```python
from build123d import *

# Parameters (mm, degrees)
SKETCH_1_R            = 12
EXTRUDE_1_DEPTH       = 55
CUT_EXTRUDE_START     = 19.5
SKETCH_2_OUTSIDE_W    = 38.926
SKETCH_2_OUTSIDE_H    = 38.926
SKETCH_2_OUTSIDE_R    = 10
CUT_EXTRUDE_1_DEPTH   = 3
SKETCH_3_R            = 11.5
EXTRUDE_2_DEPTH       = 18
SKETCH_4_OUTSIDE_W    = 42.1
SKETCH_4_OUTSIDE_H    = 42.1
SKETCH_4_OUTSIDE_R    = 11
CUT_EXTRUDE_2_DEPTH   = 2.5
SKETCH_5_R            = 10
EXTRUDE_3_DEPTH       = 16
SKETCH_6_OUTSIDE_W    = 45.05
SKETCH_6_OUTSIDE_H    = 45.05
SKETCH_6_OUTSIDE_R    = 9.5
CUT_EXTRUDE_3_DEPTH   = 2.5
SKETCH_7_R            = 9.5
EXTRUDE_4_DEPTH       = 28
SKETCH_9_R            = 10
EXTRUDE_6_DEPTH       = 15
SKETCH_10_R           = 10
EXTRUDE_7_DEPTH       = 24
SKETCH_11_OUTSIDE_W   = 57.93
SKETCH_11_OUTSIDE_H   = 57.93
SKETCH_11_OUTSIDE_R   = 9
CUT_EXTRUDE_4_DEPTH   = 11
CUT_EXTRUDE_START_2   = -21.5
SKETCH_12_OUTSIDE_W   = 57.93
SKETCH_12_OUTSIDE_H   = 57.93
SKETCH_12_OUTSIDE_R   = 9
CUT_EXTRUDE_5_DEPTH   = 2.5
CUT_EXTRUDE_8_DEPTH   = 157.920361967
CUT_EXTRUDE_START_3   = 8
CUT_EXTRUDE_9_DEPTH   = 149.920361967
CUT_EXTRUDE_START_4   = 8.5
CUT_EXTRUDE_10_DEPTH  = 149.420361967
F_2_0MM_1_D           = 2
F_2_0MM_1_DEPTH       = 5
F_2_0MM_1_CSINK_D     = 5
F_2_0MM_1_CSINK_ANGLE = 60
F_2_0MM_1_TIP         = 0.600860619
F_2_0MM_4_D           = 2
F_2_0MM_4_DEPTH       = 5
F_2_0MM_4_CSINK_D     = 5
F_2_0MM_4_CSINK_ANGLE = 60
F_2_0MM_4_TIP         = 0.600860619


# Read off the part's stored shape, not the designer's step: M20 机械螺纹 螺柱1
with BuildPart() as part:
    # 草图1 → 凸台-拉伸1 (new body)
    with BuildSketch(Plane.XY):
        Circle(SKETCH_1_R)
    extrude(amount=EXTRUDE_1_DEPTH)

    # 草图2 outside → 切除-拉伸1 (cut)
    with BuildSketch(Plane.XY.offset(CUT_EXTRUDE_START)):
        Rectangle(SKETCH_2_OUTSIDE_W, SKETCH_2_OUTSIDE_H)
        Circle(SKETCH_2_OUTSIDE_R, mode=Mode.SUBTRACT)
    extrude(amount=CUT_EXTRUDE_1_DEPTH, mode=Mode.SUBTRACT)

    # 草图3 → 凸台-拉伸2 (add)
    with BuildSketch(Plane.XY.offset(55)):
        Circle(SKETCH_3_R)
    extrude(amount=EXTRUDE_2_DEPTH)

    # 草图4 outside → 切除-拉伸2 (cut)
    with BuildSketch(Plane.XY.offset(55)):
        Rectangle(SKETCH_4_OUTSIDE_W, SKETCH_4_OUTSIDE_H)
        Circle(SKETCH_4_OUTSIDE_R, mode=Mode.SUBTRACT)
    extrude(amount=CUT_EXTRUDE_2_DEPTH, mode=Mode.SUBTRACT)

    # 草图5 → 凸台-拉伸3 (add)
    with BuildSketch(Plane.XY.offset(73)):
        Circle(SKETCH_5_R)
    extrude(amount=EXTRUDE_3_DEPTH)

    # 草图6 outside → 切除-拉伸3 (cut)
    with BuildSketch(Plane.XY.offset(73)):
        Rectangle(SKETCH_6_OUTSIDE_W, SKETCH_6_OUTSIDE_H)
        Circle(SKETCH_6_OUTSIDE_R, mode=Mode.SUBTRACT)
    extrude(amount=CUT_EXTRUDE_3_DEPTH, mode=Mode.SUBTRACT)

    # 草图7 → 凸台-拉伸4 (add)
    with BuildSketch(Plane.XY.offset(89)):
        Circle(SKETCH_7_R)
    extrude(amount=EXTRUDE_4_DEPTH)

    # 草图9 → 凸台-拉伸6 (add)
    with BuildSketch(Plane.XY.offset(117)):
        Circle(SKETCH_9_R)
    extrude(amount=EXTRUDE_6_DEPTH)

    # 草图10 → 凸台-拉伸7 (add)
    with BuildSketch(Plane.XY.offset(132)):
        Circle(SKETCH_10_R)
    extrude(amount=EXTRUDE_7_DEPTH)

    # 草图11 outside → 切除-拉伸4 (cut)
    with BuildSketch(Plane.XY.offset(156)):
        Rectangle(SKETCH_11_OUTSIDE_W, SKETCH_11_OUTSIDE_H)
        Circle(SKETCH_11_OUTSIDE_R, mode=Mode.SUBTRACT)
    extrude(amount=-CUT_EXTRUDE_4_DEPTH, mode=Mode.SUBTRACT)

    # 草图12 outside → 切除-拉伸5 (cut)
    with BuildSketch(Plane.XY.offset(156).offset(CUT_EXTRUDE_START_2)):
        Rectangle(SKETCH_12_OUTSIDE_W, SKETCH_12_OUTSIDE_H)
        Circle(SKETCH_12_OUTSIDE_R, mode=Mode.SUBTRACT)
    extrude(amount=-CUT_EXTRUDE_5_DEPTH, mode=Mode.SUBTRACT)

    # M20 机械螺纹 螺柱1 outline → M20 机械螺纹 螺柱1 (revolve, cut)
    with BuildSketch(Plane.XZ):
        Polygon((10, 145), (8.647, 145), (10, 143.647), align=None)
    revolve(axis=Axis((0, 0, 0), (0, 0, 1)), mode=Mode.SUBTRACT)

    # 草图14 → 切除-拉伸8 (cut, symmetric)
    with BuildSketch(Plane(origin=(0, 0, 0), x_dir=(0, 0, -1), z_dir=(1, 0, 0))):
        Polygon((-479.636732543, 4), (-156, 4), (-145, 4), (-145, 14.592114555), (-145, 338.228847098), (-602.412263469, 796.199326311), (-937.048996012, 461.970479214), align=None)
    cut_extrude_8 = extrude(amount=CUT_EXTRUDE_8_DEPTH, both=True, mode=Mode.SUBTRACT)

    # 镜向1: 切除-拉伸8 across plane
    add(cut_extrude_8.mirror(Plane.ZX), mode=Mode.SUBTRACT)

    # 草图15 → 切除-拉伸9 (cut, through all)
    with BuildSketch(Plane(origin=(0, 0, 0), x_dir=(1, 0, 0), z_dir=(0, 1, 0)).offset(CUT_EXTRUDE_START_3)):
        with BuildLine():
            Line((-3, -145), (-3, -131))
            ThreePointArc((-3, -131), (0, -128), (3, -131))
            Line((3, -131), (3, -145))
            ThreePointArc((3, -145), (0, -148), (-3, -145))
        make_face()
    extrude(amount=CUT_EXTRUDE_9_DEPTH, mode=Mode.SUBTRACT)

    # 草图17 → 切除-拉伸10 (cut, through all)
    with BuildSketch(Plane(origin=(0, 0, 0), x_dir=(1, 0, 0), z_dir=(0, 1, 0)).offset(CUT_EXTRUDE_START_4)):
        with BuildLine():
            Line((3, -4.5), (3, -14.5))
            ThreePointArc((3, -14.5), (0, -17.5), (-3, -14.5))
            Line((-3, -14.5), (-3, -4.5))
            ThreePointArc((-3, -4.5), (0, -1.5), (3, -4.5))
        make_face()
    extrude(amount=CUT_EXTRUDE_10_DEPTH, mode=Mode.SUBTRACT)

    # Ø2.0mm 暗销孔1
    with Locations(Plane(origin=(0, 0, 0), x_dir=(-1, 0, 0), z_dir=(0, 0, -1))):
        with Locations((0, 0)):
            CounterSinkHole(F_2_0MM_1_D / 2, F_2_0MM_1_CSINK_D / 2, depth=F_2_0MM_1_DEPTH, counter_sink_angle=F_2_0MM_1_CSINK_ANGLE)
            with Locations((0, 0, -(F_2_0MM_1_DEPTH + F_2_0MM_1_TIP / 2))):  # 118° drill point
                Cone(0, F_2_0MM_1_D / 2, F_2_0MM_1_TIP, mode=Mode.SUBTRACT)

    # Ø2.0mm 暗销孔4
    with Locations(Plane.XY.offset(156)):
        with Locations((0, 0)):
            CounterSinkHole(F_2_0MM_4_D / 2, F_2_0MM_4_CSINK_D / 2, depth=F_2_0MM_4_DEPTH, counter_sink_angle=F_2_0MM_4_CSINK_ANGLE)
            with Locations((0, 0, -(F_2_0MM_4_DEPTH + F_2_0MM_4_TIP / 2))):  # 118° drill point
                Cone(0, F_2_0MM_4_D / 2, F_2_0MM_4_TIP, mode=Mode.SUBTRACT)


solid = part.part
```
Part model, mm, in its own coordinate system. A direction names the side the tool comes from. Round coordinates to 2 decimals unless told otherwise and drop trailing zeros. Order: outer loops, then holes, each group sorted by start corner. A loop starts at its lowest first (then second) coordinate and runs counter-clockwise, first axis right, second up. Notation, with made-up numbers: M -7,32.5 L 43,32.5 A37 cw 43,70.5 Z; hole C 25.25,23.5 d7. An arc over 180 degrees is marked long. Put each result on its own line as item: value. Start each with the question number.
1. Two-plate mould, pull along X, no slides. Class faces 4 (the face through (-3, 10, 10)), 5 (the face through (-2, -9, 134.5)), 6 (the face through (0, -9, 133)): +X half, -X half, draft (parallel to the pull), parting line (faces both ways), or undercut.
2. Drill centre lines: probe 1 along Y at (x, z) = (0, 3.5); probe 2 along Y at (x, z) = (0, 152.8); probe 3 along X at (y, z) = (0, 151.85). Where is each one in solid material? Low to high. Write a range as [from, to].
3. Slice it at A-A on z = 141.5. List the corners of the cut face in (x, y), then the cut area to 3 significant figures.
4. Drop flat-ended pins along their axis: pin 1 (7 mm diameter, centred on x = -5, y = 5.5, fed in from -Z); pin 2 (1.8 mm diameter, centred on x = 1, z = 140, fed in from +Y); pin 3 (2.5 mm diameter, centred on x = 2, y = -5.5, fed in from +Z); pin 4 (3 mm diameter, centred on y = 6, z = 119, fed in from -X). Give the stop position or say it passes through.
5. Tool access for faces 1 (the face through (4.38, -8.43, 102.8)), 2 (the face through (0, -4, 151)), 3 (the face through (0, 6, 145)): list every direction of +Z, -Z, +X, -X, +Y, -Y with a clear straight run to the whole face (end or side of a thin tool).
Findings:
1. face 4: undercut
1. face 5: draft
1. face 6: parting line
2. probe 1: [-12, -1], [1, 8.5]
2. probe 2: [-4, -1], [1, 4]
2. probe 3: [-9, -1], [1, 9]
3. outline: M -3,8 L -3,9.54 A10 ccw long 3,9.54 L 3,8 Z
3. area: 303 mm2
4. pin 1: z = 0
4. pin 2: y = 8
4. pin 3: z = 145
4. pin 4: x = -8.93
5. face 1: none
5. face 2: +Z, +X, -X, -Y
5. face 3: +Z, +X, -X, +Y
